Work out the finished part from the listing and answer in its coordinate system (mm). Face numbers are marked on the shaded views. A direction names the side the tool comes from. Round coordinates to 2 decimals unless told otherwise and drop trailing zeros. Loops run counter-clockwise (first coordinate to the right, second up) from the corner with the lowest first, then second, coordinate; pieces in that order, holes last. Notation, with made-up numbers: (22, -24) - (78, -24) arc R21 cw to (78, -16) - close; hole circle Ø6 at (-3, 33.25). An arc over 180 degrees is marked (long way). Answer as CSV lines item,"result". Start each with the question number.
Q1. Section C-C on z = 58 is taken. Write down the section's boundary in (x, y), then the cut area to 3 significant figures.
Q2. Section A-A on x = -245 is taken. Write down the section's boundary in (y, z), then the cut area to 4 significant figures.
Q3. Section B-B on y = -35 is taken. Write down the section's boundary in (x, z), then the cut area to 3 significant figures.
Q4. This flat-tipped pin is pushed along its axis until it touches: pin 1 Ø4 at (y, z) = (-43.5, 70.5) entering from +X. Where does it stop, or does it pass through?
Q5. For the marked faces 4 and 5, determine the directions among +Z, -Z, +X, -X, +Y, -Y from which every point of the face is accessible in a straight line to the end or side of a thin tool.
Q6. Straight lines are drawn through the part: L1, parallel to Z at x = -248.5, y = -11; L2, parallel to Y at x = -245, z = 63.5. For each, find the intervals that lie inside material, in ascending order. Write a range as [from, to].
Q7. The mould has two halves that part along Z. Classify the marked faces 1, 2 and 3: +Z half, -Z half, draft (parallel to the pull), parting line (faces both ways), or undercut.
```python
from build123d import *

# Parameters (mm, degrees)
MAIN_PROFILE_SKETCH_W   = 31.5
MAIN_PROFILE_SKETCH_H   = 44
MAIN_PROFILE_SKETCH_W_2 = 28.5
MAIN_PROFILE_SKETCH_H_2 = 41
MAIN_EXTRUSION_DEPTH    = 10


with BuildPart() as part:
    # Main Profile Sketch → Main Extrusion (new body)
    with BuildSketch(Plane(origin=(-240, 0, 0), x_dir=(0, 0, -1), z_dir=(1, 0, 0))):
        with Locations((-64.25, -26.5)):
            Rectangle(MAIN_PROFILE_SKETCH_W, MAIN_PROFILE_SKETCH_H)
        with Locations((-64.25, -26.5)):
            Rectangle(MAIN_PROFILE_SKETCH_W_2, MAIN_PROFILE_SKETCH_H_2, mode=Mode.SUBTRACT)
    extrude(amount=-MAIN_EXTRUSION_DEPTH)


solid = part.part
```
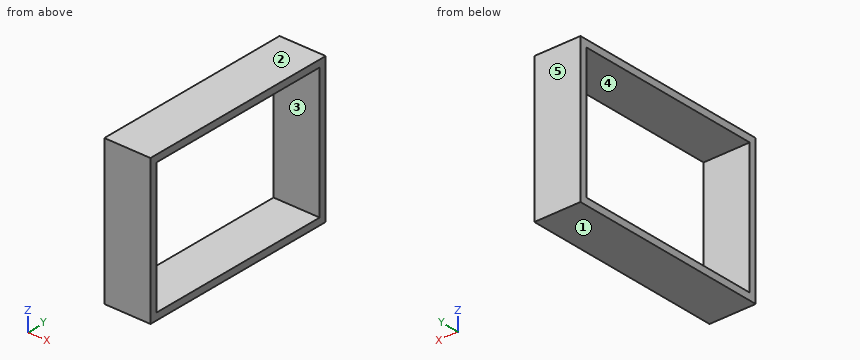
Findings:
1,outline,"(-250, -48.5) - (-240, -48.5) - (-240, -47) - (-250, -47) - close; (-250, -6) - (-240, -6) - (-240, -4.5) - (-250, -4.5) - close"
1,area,"30.0 mm^2"
2,outline,"(-48.5, 48.5) - (-4.5, 48.5) - (-4.5, 80) - (-48.5, 80) - close; hole (-47, 50) - (-6, 50) - (-6, 78.5) - (-47, 78.5) - close"
2,area,"217.5 mm^2"
3,outline,"(-250, 48.5) - (-240, 48.5) - (-240, 50) - (-250, 50) - close; (-250, 78.5) - (-240, 78.5) - (-240, 80) - (-250, 80) - close"
3,area,"30.0 mm^2"
4,pin 1,"passes through"
5,face 4,"+X, -X"
5,face 5,"+Z, -Z, +X, -X, +Y"
6,L1,"z = [48.5, 50], [78.5, 80]"
6,L2,"y = [-48.5, -47], [-6, -4.5]"
7,face 1,"-Z half"
7,face 2,"+Z half"
7,face 3,"undercut"
